from build123d import *

# Parameters (mm, degrees)
SKETCH1_W            = 92.135626016
SKETCH1_H            = 40
BOSS_EXTRUDE2_DEPTH  = 10
SKETCH2_R            = 1.5
BOSS_EXTRUDE3_DEPTH  = 1.6
SKETCH3_R            = 1
CUT_EXTRUDE1_DEPTH   = 2
SKETCH4_W            = 100.5
SKETCH4_H            = 62.5
SKETCH4_W_2          = 98.5
SKETCH4_H_2          = 60.5
BOSS_EXTRUDE4_DEPTH  = 19.65
SKETCH5_W            = 98
SKETCH5_H            = 40
CUT_EXTRUDE5_DEPTH   = 14.65
SKETCH6_W            = 98.5
SKETCH6_H            = 10.25
BOSS_EXTRUDE5_DEPTH  = 10
SKETCH7_W            = 0.6
SKETCH7_H            = 40.584325063
BOSS_EXTRUDE11_DEPTH = 4
SKETCH8_W            = 0.6
SKETCH8_H            = 40
BOSS_EXTRUDE12_DEPTH = 4
FILLET1_R            = 1
CUT_EXTRUDE6_DEPTH   = 4
SKETCH10_W           = 1
SKETCH10_H           = 2.5
CUT_EXTRUDE8_DEPTH   = 4


with BuildPart() as part:
    # Sketch1 → Boss-Extrude2 (new body)
    with BuildSketch(Plane(origin=(0, 0, 0), x_dir=(0, 0, -1), z_dir=(1, 0, 0))):
        Polygon((-40.481927711, 26.144578313), (-43.416301695, 26.144578313), (-43.416301695, -33.855421687), (-40.481927711, -33.855421687), (54.583698305, -33.855421687), (54.583698305, 26.144578313), (33.734939759, 26.144578313), align=None)
        with Locations((5.585885297, -3.855421687)):
            Rectangle(SKETCH1_W, SKETCH1_H, mode=Mode.SUBTRACT)
    extrude(amount=BOSS_EXTRUDE2_DEPTH)

    # Sketch2 → Boss-Extrude3 (add)
    with BuildSketch(Plane(origin=(10, 0, 0), x_dir=(0, 0, -1), z_dir=(1, 0, 0))):
        with Locations((-40.916301695, 23.644578313)):
            Circle(SKETCH2_R)
        with Locations(Location((52.083698305, 23.644578313, 0), (0, 0, 180))):
            Circle(SKETCH2_R)
        with Locations((52.083698305, -31.355421687)):
            Circle(SKETCH2_R)
        with Locations(Location((-40.916301695, -31.355421687, 0), (0, 0, 180))):
            Circle(SKETCH2_R)
    extrude(amount=BOSS_EXTRUDE3_DEPTH)

    # Sketch3 → Cut-Extrude1 (cut)
    with BuildSketch(Plane(origin=(11.6, 0, 0), x_dir=(0, 0, -1), z_dir=(1, 0, 0))):
        with Locations((-40.916301695, 23.644578313)):
            Circle(SKETCH3_R)
        with Locations((52.083698305, 23.644578313)):
            Circle(SKETCH3_R)
        with Locations((52.083698305, -31.355421687)):
            Circle(SKETCH3_R)
        with Locations((-40.916301695, -31.355421687)):
            Circle(SKETCH3_R)
    extrude(amount=-CUT_EXTRUDE1_DEPTH, mode=Mode.SUBTRACT)

    # Sketch5 → Cut-Extrude5 (cut)
    with BuildSketch(Plane.ZY):
        with Locations((-5.583698305, -3.855421687)):
            Rectangle(SKETCH5_W, SKETCH5_H)
    extrude(amount=-CUT_EXTRUDE5_DEPTH, mode=Mode.SUBTRACT)


with BuildPart() as body_2:
    # Sketch4 → Boss-Extrude4 (new body)
    with BuildSketch(Plane.ZY):
        with Locations((-5.583698305, -3.855421687)):
            Rectangle(SKETCH4_W, SKETCH4_H)
        with Locations((-5.583698305, -3.855421687)):
            Rectangle(SKETCH4_W_2, SKETCH4_H_2, mode=Mode.SUBTRACT)
    extrude(amount=-BOSS_EXTRUDE4_DEPTH)



with BuildPart() as cut_extrude5_piece_1:
    # of the separate pieces the step leaves, piece 1, a body of its own (cut_extrude5_pieces)
    add(part.part.solids().sort_by_distance((0, 26.144578313, -54.583698305))[0])


with BuildPart() as cut_extrude5_piece_2:
    # of the separate pieces the step leaves, piece 2, a body of its own (cut_extrude5_pieces)
    add(part.part.solids().sort_by_distance((0, -23.855421687, 43.416301695))[0])


with BuildPart() as body_2_1:
    add(body_2.part)

    add(cut_extrude5_piece_1.part)  # Boss-Extrude5 merges Cut-Extrude5 piece 1

    add(cut_extrude5_piece_2.part)  # Boss-Extrude5 merges Cut-Extrude5 piece 2
    # Sketch6 → Boss-Extrude5 (add)
    with BuildSketch(Plane.ZY):
        with Locations((-5.583698305, 21.269578313)):
            Rectangle(SKETCH6_W, SKETCH6_H)
        with Locations((-5.583698305, -28.980421687)):
            Rectangle(SKETCH6_W, SKETCH6_H)
    extrude(amount=-BOSS_EXTRUDE5_DEPTH)

    # Sketch7 → Boss-Extrude11 (add)
    with BuildSketch(Plane.ZY):
        with Locations((-54.533698305, -4.147584219)):
            Rectangle(SKETCH7_W, SKETCH7_H)
    extrude(amount=-BOSS_EXTRUDE11_DEPTH)

    # Sketch8 → Boss-Extrude12 (add)
    with BuildSketch(Plane.ZY):
        with Locations((43.366301695, -3.855421687)):
            Rectangle(SKETCH8_W, SKETCH8_H)
    extrude(amount=-BOSS_EXTRUDE12_DEPTH)

    # Fillet1
    fillet1_edges = [body_2_1.edges().sort_by_distance(p)[0] for p in [
        (0, 27.394578313, -5.583698305),
        (0, -3.855421687, 44.666301695),
        (0, -35.105421687, -5.583698305),
        (0, -3.855421687, -55.833698305),
    ]]
    fillet(fillet1_edges, radius=FILLET1_R)

    # Sketch9 → Cut-Extrude6 (cut)
    with BuildSketch(Plane(origin=(19.65, 0, 0), x_dir=(0, 0, -1), z_dir=(1, 0, 0))):
        Polygon((54.833698305, 22.144578313), (47.033698305, 22.144578313), (47.033698305, 12.024578313), (54.833698305, 12.024578313), (55.833698305, 12.024578313), (55.833698305, 22.144578313), align=None)
    extrude(amount=-CUT_EXTRUDE6_DEPTH, mode=Mode.SUBTRACT)

    # Sketch10 → Cut-Extrude8 (cut)
    with BuildSketch(Plane(origin=(19.65, 0, 0), x_dir=(0, 0, -1), z_dir=(1, 0, 0))):
        with Locations((55.333698305, 10.774578313)):
            Rectangle(SKETCH10_W, SKETCH10_H)
    extrude(amount=-CUT_EXTRUDE8_DEPTH, mode=Mode.SUBTRACT)


solid = body_2_1.part
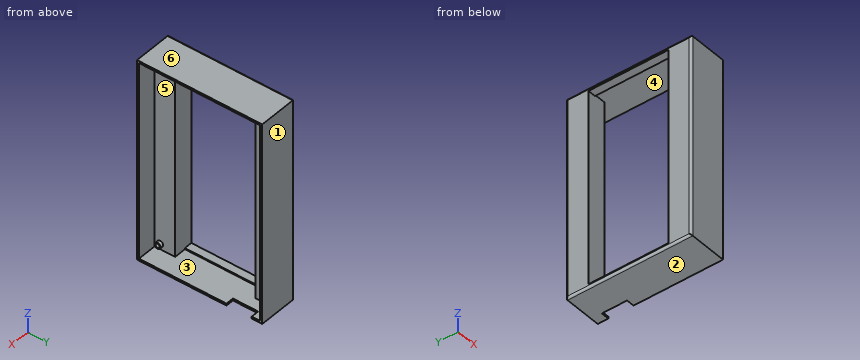
Geometry check sheet. Reference: the model listing, model coordinates, mm. Face numbers are marked on the shaded views. A direction names the side the tool comes from. Give positions to 0.01 mm unless a question says otherwise; leave off trailing zeros. Loops run counter-clockwise (first coordinate to the right, second up) from the corner with the lowest first, then second, coordinate; pieces in that order, holes last.
(1) Section check C-C on x = 8. Record the cut outline in (y, z).
From the geometry:
outline: (-35.11, -55.83) - (27.39, -55.83) - (27.39, 44.67) - (-35.11, 44.67) - close; hole (-23.86, -54.83) - (16.14, -54.83) - (16.14, 43.67) - (-23.86, 43.67) - close
(2) Section check A-A on z = 35. Record the cut outline in (x, y), then the cut area to 3 significant figures.
From the geometry:
outline: (0, -34.11) arc R1 ccw to (1, -35.11) - (19.65, -35.11) - (19.65, -34.11) - (10, -34.11) - (10, -23.86) - (0, -23.86) - close; (0, 16.14) - (10, 16.14) - (10, 26.39) - (19.65, 26.39) - (19.65, 27.39) - (1, 27.39) arc R1 ccw to (0, 26.39) - close
area: 244 mm2
(3) Section check D-D on x = 17.75. Record the cut outline in (y, z).
From the geometry:
outline: (-35.11, -55.83) - (9.52, -55.83) - (9.52, -54.83) - (-34.11, -54.83) - (-34.11, 43.67) - (26.39, 43.67) - (26.39, -54.83) - (22.14, -54.83) - (22.14, -55.83) - (27.39, -55.83) - (27.39, 44.67) - (-35.11, 44.67) - close
(4) Set-up check for the marked faces 5 and 6: record each of +Z, -Z, +X, -X, +Y, -Y from which the full face is reachable in a straight line by a thin tool's end or side.
From the geometry:
face 5: +X
face 6: +Z, +X, -X, +Y, -Y
(5) Release check for a two-part mould opening along Y. For the marked faces 1, 2, 3 and 4 record: released by +Y, released by -Y, zero draft, split by the parting line, or undercut.
From the geometry:
face 1: released by +Y
face 2: zero draft
face 3: undercut
face 4: undercut
(6) Section check B-B on y = 0. Record the cut outline in (x, z).
From the geometry:
outline: (0, -54.83) arc R1 ccw to (1, -55.83) - (19.65, -55.83) - (19.65, -54.83) - (4, -54.83) - (4, -54.23) - (0, -54.23) - close; (0, 43.07) - (4, 43.07) - (4, 43.67) - (19.65, 43.67) - (19.65, 44.67) - (1, 44.67) arc R1 ccw to (0, 43.67) - close
(7) Thickness scan on L1, parallel to Y at x = 13, z = 35; L2, parallel to Z at x = 4.5, y = -1; L3, parallel to Y at x = 1, z = -33.5. Record the ranges inside material, lowest first.
From the geometry:
L1: y = -35.11 to -34.11, 26.39 to 27.39
L2: z = -55.83 to -54.83, 43.67 to 44.67
L3: y = -35.11 to -23.86, 16.14 to 27.39
(8) Depth check by flat-ended pin: pin 1 Ø8 at (y, z) = (19.5, -22.5) entering from +X; pin 2 Ø1.5 at (y, z) = (-32, -52) entering from +X. Enter the tip coordinate at first touch or a pass-through.
From the geometry:
pin 1: stops at x = 10
pin 2: stops at x = 11.6
